Read the model definition and answer for the solid it produces. Units are mm, in the model's axes. Coordinates: 2 decimals unless noted, no trailing zeros. Loops run counter-clockwise (first coordinate to the right, second up) from the corner with the lowest first, then second, coordinate; pieces in that order, holes last.
Q1. A flat-ended cylindrical pin translates along its axis: P1, Ø5, axis at x = -16, z = 22, coming from the +Y side. Find the tip coordinate at first contact, or state that the pin passes through.
Q2. Straight lines are drawn through the part: line 1 (X direction, y = -3.75, z = 22); line 2 (X direction, y = 2.5, z = 6); line 3 (Y direction, x = 18, z = 19). For each, find the intervals that lie inside material, in ascending order.
Q3. Section A-A (y = 0) is taken. Give the vertices of the cut face in (x, z), then the cut area to 3 significant figures.
Q4. Section C-C (z = 14) is taken. Give the vertices of the cut face in (x, y), then the cut area to 3 significant figures.
Q5. Section D-D (y = -8.5) is taken. Give the vertices of the cut face in (x, z).
Q6. The mould has two halves that part along Y. Classify faces 1 (the face through (27.3, 2.93, 14.79)), 2 (the face through (-10, 6, 15)), 3 (the face through (0, 0, 30)): pulls with the +Y half, pulls with the -Y half, needs draft (parallel to the pull), parting line crosses it, or undercut.
Q7. Section B-B (x = 18) is taken. Give the vertices of the cut face in (y, z), then the cut area to 3 significant figures.
from build123d import *
from build123d.topology import SkipClean

# Parameters (mm, degrees)
SKETCH1_W           = 60
SKETCH1_H           = 25
SKETCH1_R           = 9.75
SKETCH1_R_2         = 5.35
BOSS_EXTRUDE1_DEPTH = 30
BOSS_EXTRUDE2_DEPTH = 0.0001
CUT_EXTRUDE1_START  = -6.5
SKETCH2_3_R         = 17.75
CUT_EXTRUDE1_DEPTH  = 6.5


with BuildPart() as part:
    # Sketch1 → Boss-Extrude1 (new body)
    with BuildSketch(Plane.XY):
        Rectangle(SKETCH1_W, SKETCH1_H)
        with Locations((18, 0)):
            Circle(SKETCH1_R, mode=Mode.SUBTRACT)
        with Locations((-22, 0)):
            Circle(SKETCH1_R_2, mode=Mode.SUBTRACT)
    extrude(amount=BOSS_EXTRUDE1_DEPTH)

    # Sketch2 → Boss-Extrude2 (add)
    with BuildSketch(Plane(origin=(0, 12.5, 0), x_dir=(1, 0, 0), z_dir=(0, 1, 0))):
        with BuildLine():
            ThreePointArc((-19.490126448, -30), (-27.75, -15), (-19.490126448, 0))
            Line((-19.490126448, 0), (-30, 0))
            Line((-30, 0), (-30, -30))
            Line((-30, -30), (-19.490126448, -30))
        make_face()
        with BuildLine():
            ThreePointArc((-0.509873552, 0), (5.548508682, -6.438085624), (7.75, -15))
            ThreePointArc((7.75, -15), (5.548508682, -23.561914376), (-0.509873552, -30))
            Line((-0.509873552, -30), (30, -30))
            Line((30, -30), (30, 0))
            Line((30, 0), (-0.509873552, 0))
        make_face()
    extrude(amount=BOSS_EXTRUDE2_DEPTH)

    # Sketch2_3 → Cut-Extrude1 (cut)
    with SkipClean():  # the faces are left unmerged after this step: merging them gives an invalid solid
        with BuildSketch(Plane(origin=(0, 12.5, 0), x_dir=(1, 0, 0), z_dir=(0, 1, 0)).offset(CUT_EXTRUDE1_START)):
            with Locations((-10, -15)):
                Circle(SKETCH2_3_R)
        extrude(amount=CUT_EXTRUDE1_DEPTH, mode=Mode.SUBTRACT)


solid = part.part
Numbers:
1. P1: stops at y = 6
2. line 1: x = -30 to -25.82, -18.18 to 9, 27 to 30
2. line 2: x = -30 to -26.73, -17.27 to 8.58, 27.42 to 30
2. line 3: y = -12.5 to -9.75, 9.75 to 12.5
3. outline: (-30, 0) - (-27.35, 0) - (-27.35, 30) - (-30, 30) - close; (-16.65, 0) - (8.25, 0) - (8.25, 30) - (-16.65, 30) - close; (27.75, 0) - (30, 0) - (30, 30) - (27.75, 30) - close
3. area: 894 mm2
4. outline: (-30, -12.5) - (30, -12.5) - (30, 12.5) - (7.72, 12.5) - (7.72, 6) - (-27.72, 6) - (-27.72, 12.5) - (-30, 12.5) - close; hole circle Ø10.7 at (-22, 0); hole circle Ø19.5 at (18, 0)
4. area: 881 mm2
5. outline: (-30, 0) - (13.22, 0) - (13.22, 30) - (-30, 30) - close; (22.78, 0) - (30, 0) - (30, 30) - (22.78, 30) - close
6. face 1: undercut
6. face 2: pulls with the +Y half
6. face 3: needs draft
7. outline: (-12.5, 0) - (-9.75, 0) - (-9.75, 30) - (-12.5, 30) - close; (9.75, 0) - (12.5, 0) - (12.5, 30) - (9.75, 30) - close
7. area: 165 mm2
